```python
from build123d import *

# Parameters (mm, degrees)
SKETCH_5_R          = 4
CUT_EXTRUDE_1_DEPTH = 55.27706698
CUT_EXTRUDE_2_DEPTH = 55.27706698
SKETCH_8_R          = 11.25
CUT_EXTRUDE_3_DEPTH = 55.27706698


with BuildPart() as part:
    # 草图3 → 旋转1 (revolve)
    with BuildSketch(Plane(origin=(0, 0, 0), x_dir=(0, 0, -1), z_dir=(1, 0, 0)), mode=Mode.PRIVATE) as revolve_1_sk:
        Polygon((0, 211.239142824), (11.25, 211.239142824), (21, 217.739142824), (31, 219.239142824), (31, 187.239142824), (0, 187.239142824), align=None)
    revolve(revolve_1_sk.sketch.rotate(Axis((0, 291.944884017, 0), (0, -1, 0)), 180), axis=Axis((0, 291.944884017, 0), (0, -1, 0)))

    # 草图5 → 切除-拉伸1 (cut, through all)
    with BuildSketch(Plane.XZ.offset(-187.239142824)):
        with Locations(Location((0, 0, 0), (0, 0, 270))):
            Circle(SKETCH_5_R)
    extrude(amount=-CUT_EXTRUDE_1_DEPTH, mode=Mode.SUBTRACT)

    # 草图6 → 切除-拉伸2 (cut, through all)
    with BuildSketch(Plane.XZ.offset(-187.239142824)):
        with BuildLine():
            ThreePointArc((-12.727922061, 12.727922061), (-9.475230868, 12.727922061), (-9.475230868, 9.475230868))
            ThreePointArc((-9.475230868, 9.475230868), (-13.048964597, 6.79154607), (-17.229268429, 5.210787791))
            ThreePointArc((-17.229268429, 5.210787791), (-15.442964172, 9.247424375), (-12.727922061, 12.727922061))
        make_face()
        with BuildLine():
            ThreePointArc((0, 18), (2.3, 15.7), (0, 13.4))
            ThreePointArc((0, 13.4), (-4.424663073, 14.029359635), (-8.498349158, 15.867515924))
            ThreePointArc((-8.498349158, 15.867515924), (-4.380908204, 17.458741172), (0, 18))
        make_face()
        with BuildLine():
            ThreePointArc((12.727922061, 12.727922061), (12.727922061, 9.475230868), (9.475230868, 9.475230868))
            ThreePointArc((9.475230868, 9.475230868), (6.79154607, 13.048964597), (5.210787791, 17.229268429))
            ThreePointArc((5.210787791, 17.229268429), (9.247424375, 15.442964172), (12.727922061, 12.727922061))
        make_face()
        with BuildLine():
            ThreePointArc((18, 0), (15.7, -2.3), (13.4, 0))
            ThreePointArc((13.4, 0), (14.029359635, 4.424663073), (15.867515924, 8.498349158))
            ThreePointArc((15.867515924, 8.498349158), (17.458741172, 4.380908204), (18, 0))
        make_face()
        with BuildLine():
            ThreePointArc((12.727922061, -12.727922061), (9.475230868, -12.727922061), (9.475230868, -9.475230868))
            ThreePointArc((9.475230868, -9.475230868), (13.048964597, -6.79154607), (17.229268429, -5.210787791))
            ThreePointArc((17.229268429, -5.210787791), (15.442964172, -9.247424375), (12.727922061, -12.727922061))
        make_face()
        with BuildLine():
            ThreePointArc((0, -18), (-2.3, -15.7), (0, -13.4))
            ThreePointArc((0, -13.4), (4.424663073, -14.029359635), (8.498349158, -15.867515924))
            ThreePointArc((8.498349158, -15.867515924), (4.380908204, -17.458741172), (0, -18))
        make_face()
        with BuildLine():
            ThreePointArc((-12.727922061, -12.727922061), (-12.727922061, -9.475230868), (-9.475230868, -9.475230868))
            ThreePointArc((-9.475230868, -9.475230868), (-6.79154607, -13.048964597), (-5.210787791, -17.229268429))
            ThreePointArc((-5.210787791, -17.229268429), (-9.247424375, -15.442964172), (-12.727922061, -12.727922061))
        make_face()
        with BuildLine():
            ThreePointArc((-13.4, 0), (-14.029359635, -4.424663073), (-15.867515924, -8.498349158))
            ThreePointArc((-15.867515924, -8.498349158), (-17.458741172, -4.380908204), (-18, 0))
            ThreePointArc((-18, 0), (-15.7, 2.3), (-13.4, 0))
        make_face()
    extrude(amount=-CUT_EXTRUDE_2_DEPTH, mode=Mode.SUBTRACT)

    # 草图8 → 切除-拉伸3 (cut, through all)
    with BuildSketch(Plane.XZ.offset(-187.239142824)):
        with Locations(Location((0, 0, 0), (0, 0, 270))):
            Circle(SKETCH_8_R)
    extrude(amount=-CUT_EXTRUDE_3_DEPTH, mode=Mode.SUBTRACT)


solid = part.part
```
Work out the finished part from the listing and answer in its coordinate system (mm). A direction names the side the tool comes from. Give positions to 0.01 mm unless a question says otherwise; leave off trailing zeros. One line per question, with ' | ' between items. Start each with the question number.
1) Section A-A, the plane y = 204 is taken. State how many separate pieces and enclosed holes the cut face has, then the cut area to 3 significant figures.
2) Each of these flat-tipped pins is pushed along its axis until it touches: pin 1 (12 mm diameter, centred on y = 202, z = 10.5, fed in from +X); pin 2 (12 mm diameter, centred on x = -6.5, y = 201, fed in from -Z); pin 3 (12 mm diameter, centred on x = -19, y = 196.5, fed in from -Z). Where does it stop, or does it pass through?
3) Straight lines are drawn through the part: L1, parallel to X at y = 202.5, z = 10; L2, parallel to X at y = 194.5, z = -11.5; L3, parallel to Z at x = 0.5, y = 204.5 (3 decimals). For each, find the intervals that lie inside material, in ascending order.
4) For faces 1 (the face through (15.75, 201.29, -2.3)), 2 (the face through (10.522, 211.646, 5.473)), determine the directions among +Z, -Z, +X, -X, +Y, -Y from which every point of the face is accessible in a straight line to the end or side of a thin tool.
Resolved:
1) separate pieces: 1 | enclosed holes: 9 | area: 2,340 mm2
2) pin 1: x = 30.67 | pin 2: z = -31 | pin 3: z = -28.14
3) L1: -29.34 to -14.97, -9.08 to -5.15, 5.15 to 8.97, 13.12 to 29.34 | L2: -28.79 to -13.37, -7.76 to 8.84, 13.85 to 28.79 | L3: -30.996 to -17.993, -13.408 to -11.239, 11.239 to 13.455, 17.945 to 30.996
4) face 1: +Y, -Y | face 2: +Y
